from build123d import *

# Parameters (mm, degrees)
SKETCH_1_W          = 330
SKETCH_1_H          = 64.5
EXTRUDE_1_DEPTH     = 1
SKETCH_2_R          = 1.6
CUT_EXTRUDE_1_DEPTH = 337.245817818
CUT_EXTRUDE_2_REACH = 338.246
SKETCH_3_W          = 25
SKETCH_3_H          = 64.5
CUT_EXTRUDE_3_REACH = 313.747


with BuildPart() as part:
    # 草图1 → 凸台-拉伸1 (new body)
    with BuildSketch(Plane(origin=(0, 0, 0), x_dir=(1, 0, 0), z_dir=(0, 1, 0))):
        with Locations((165, 32.25)):
            Rectangle(SKETCH_1_W, SKETCH_1_H)
    extrude(amount=EXTRUDE_1_DEPTH)

    # 草图2 → 切除-拉伸1 (cut, through all)
    with BuildSketch(Plane(origin=(0, 1, 0), x_dir=(1, 0, 0), z_dir=(0, 1, 0))):
        with Locations(Location((35, 61.5, 0), (0, 0, 270))):
            Circle(SKETCH_2_R)
        with Locations(Location((55, 61.5, 0), (0, 0, 270))):
            Circle(SKETCH_2_R)
        with Locations(Location((280, 61.5, 0), (0, 0, 270))):
            Circle(SKETCH_2_R)
        with Locations(Location((300, 61.5, 0), (0, 0, 270))):
            Circle(SKETCH_2_R)
        with Locations(Location((300, 3, 0), (0, 0, 90))):
            Circle(SKETCH_2_R)
        with Locations(Location((280, 3, 0), (0, 0, 90))):
            Circle(SKETCH_2_R)
        with Locations(Location((55, 3, 0), (0, 0, 90))):
            Circle(SKETCH_2_R)
        with Locations(Location((35, 3, 0), (0, 0, 90))):
            Circle(SKETCH_2_R)
        with Locations(Location((300, 37.25, 0), (0, 0, 90))):
            Circle(SKETCH_2_R)
        with Locations(Location((300, 17.25, 0), (0, 0, 90))):
            Circle(SKETCH_2_R)
        with Locations(Location((5, 5, 0), (0, 0, 270))):
            Circle(SKETCH_2_R)
    extrude(amount=-CUT_EXTRUDE_1_DEPTH, mode=Mode.SUBTRACT)

    # 草图3 → 切除-拉伸2 (cut, up to next)
    with BuildSketch(Plane(origin=(0, 1, 0), x_dir=(1, 0, 0), z_dir=(0, 1, 0)), mode=Mode.PRIVATE) as cut_extrude_2_sk1:
        with Locations((317.5, 32.25)):
            Rectangle(SKETCH_3_W, SKETCH_3_H)
    cut_extrude_2_tool1 = extrude(cut_extrude_2_sk1.sketch, amount=-CUT_EXTRUDE_2_REACH, mode=Mode.PRIVATE) & part.part
    add(cut_extrude_2_tool1.solids().sort_by_distance((317.5, 1, -32.25))[0], mode=Mode.SUBTRACT)

    # 草图4 → 切除-拉伸3 (cut, up to next)
    with BuildSketch(Plane(origin=(0, 1, 0), x_dir=(1, 0, 0), z_dir=(0, 1, 0)), mode=Mode.PRIVATE) as cut_extrude_3_sk1:
        with BuildLine():
            Line((140, 52.5), (155, 52.5))
            ThreePointArc((155, 52.5), (158, 49.5), (155, 46.5))
            Line((155, 46.5), (140, 46.5))
            ThreePointArc((140, 46.5), (137, 49.5), (140, 52.5))
        make_face()
    cut_extrude_3_tool1 = extrude(cut_extrude_3_sk1.sketch, amount=-CUT_EXTRUDE_3_REACH, mode=Mode.PRIVATE) & part.part
    # 草图4 → 切除-拉伸3 (cut, up to next)
    with BuildSketch(Plane(origin=(0, 1, 0), x_dir=(1, 0, 0), z_dir=(0, 1, 0)), mode=Mode.PRIVATE) as cut_extrude_3_sk2:
        with BuildLine():
            Line((20, 52.5), (60, 52.5))
            ThreePointArc((60, 52.5), (63, 49.5), (60, 46.5))
            Line((60, 46.5), (20, 46.5))
            ThreePointArc((20, 46.5), (17, 49.5), (20, 52.5))
        make_face()
    cut_extrude_3_tool2 = extrude(cut_extrude_3_sk2.sketch, amount=-CUT_EXTRUDE_3_REACH, mode=Mode.PRIVATE) & part.part
    add(cut_extrude_3_tool1.solids().sort_by_distance((147.5, 1, -49.5))[0], mode=Mode.SUBTRACT)
    add(cut_extrude_3_tool2.solids().sort_by_distance((40, 1, -49.5))[0], mode=Mode.SUBTRACT)


solid = part.part
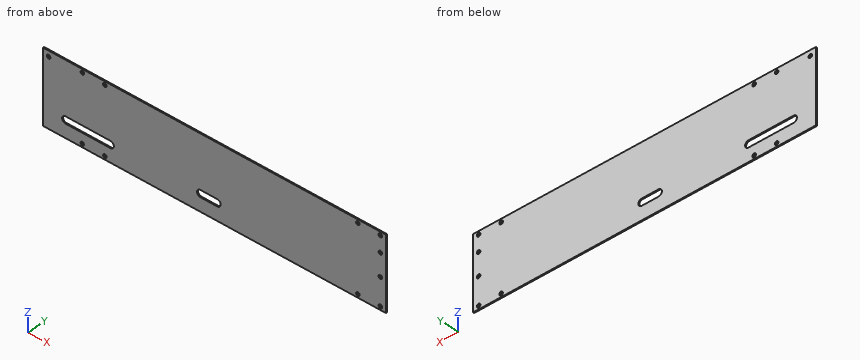
Here's how the part is built. I have some questions about the finished solid (model axes, mm). Round coordinates to 2 decimals unless told otherwise and drop trailing zeros. Write each loop counter-clockwise with the first axis right and the second up, starting at its lowest first coordinate (ties: lowest second). Pieces come first, ordered by that corner, then holes.
1. Suppose I cut it at B-B (y = 0.45). State how many separate pieces and enclosed holes the cut face has, and give its area (3 significant figures).
2. I need wall thicknesses on L1, parallel to X at y = 0.5, z = -3; L2, parallel to Z at x = 300, y = 0.65. Which ranges of each line are inside material? Lowest first, please.
3. Suppose I cut it at A-A (z = -49.5). List the corners of the cut face in (x, y) for me.
Answer sheet:
1. separate pieces: 1
1. enclosed holes: 13
1. area: 19,200 mm2
2. L1: x = 0 to 33.4, 36.6 to 53.4, 56.6 to 278.4, 281.6 to 298.4, 301.6 to 305
2. L2: z = -64.5 to -63.1, -59.9 to -38.85, -35.65 to -18.85, -15.65 to -4.6, -1.4 to 0
3. outline: (0, 0) - (17, 0) - (17, 1) - (0, 1) - close; (63, 0) - (137, 0) - (137, 1) - (63, 1) - close; (158, 0) - (305, 0) - (305, 1) - (158, 1) - close
